from build123d import *

# Parameters (mm, degrees)
SKETCH1_R           = 3.175
BOSS_EXTRUDE1_DEPTH = 12.7
SKETCH2_R           = 5.08
BOSS_EXTRUDE2_DEPTH = 3.175
MOVE_FACE1_BY       = 0.250000008


with BuildPart() as part:
    # Sketch1 → Boss-Extrude1 (new body)
    with BuildSketch(Plane.XY):
        Circle(SKETCH1_R)
    extrude(amount=BOSS_EXTRUDE1_DEPTH)

    # Sketch2 → Boss-Extrude2 (add)
    with BuildSketch(Plane(origin=(0, 0, 0), x_dir=(-1, 0, 0), z_dir=(0, 0, -1))):
        Circle(SKETCH2_R)
    extrude(amount=BOSS_EXTRUDE2_DEPTH)

    # Move Face1: a curved face moved inward by 0.25
    add(Solid.thicken(part.faces().sort_by_distance((-3.175, 0, 6.35))[0], -MOVE_FACE1_BY), mode=Mode.SUBTRACT)


solid = part.part
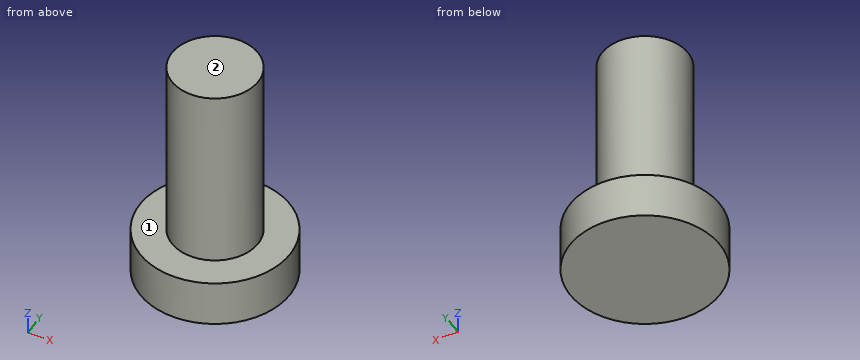
Geometry check sheet. Reference: the model listing, model coordinates, mm. Face numbers are marked on the shaded views. A direction names the side the tool comes from. Coordinates: 2 decimals unless noted, no trailing zeros. Loops run counter-clockwise (first coordinate to the right, second up) from the corner with the lowest first, then second, coordinate; pieces in that order, holes last. Notation, with made-up numbers: (62, 56.5) - (96, 56.5) arc R26 ccw to (96, 78.5) - close; hole circle Ø7 at (-7, 18). An arc over 180 degrees is marked (long way). Use one line per item in the form item = value. Start each with the question number.
Item 1: Section check D-D, the plane y = 3.5. Enter the section's corners in (x, z) (3 decimals), and give its area (3 significant figures).
Item 2: Tool access check on the marked faces 1 and 2. Record the directions out of +Z, -Z, +X, -X, +Y, -Y that give a thin tool (end or side, any length) a straight path to the whole face; none if there is none.
Item 3: Section check C-C, the plane z = 5.25. Enter the section's corners in (x, y) (3 decimals), and give its area (3 significant figures).
Item 4: Thickness scan on probe 1 along Z at (x, y) = (-0.25, 4) (3 decimals); probe 2 along X at (y, z) = (4, -1.25); probe 3 along Y at (x, z) = (2, 5.25). Record the ranges inside material, lowest first.
Item 5: Gauge pin test, flat ends, axial feed: pin 1 (6 mm diameter, centred on x = -0.5, z = 9, fed in from +Y) (3 decimals); pin 2 (5 mm diameter, centred on x = -3, z = 1.5, fed in from -Y); pin 3 (1.5 mm diameter, centred on x = 2.5, y = -3, fed in from +Z). Record the tip position at first contact, or that the pin passes through.
Item 6: Section check A-A, the plane x = 0. Enter the section's corners in (y, z) (3 decimals), and give its area (3 significant figures).
Computed:
q1.outline = (-3.682, -3.175) - (3.682, -3.175) - (3.682, 0) - (-3.682, 0) - close
q1.area = 23.4 mm2
q2.face_1 = +Z
q2.face_2 = +Z, +X, -X, +Y, -Y
q3.outline = circle Ø5.85 at (0, 0)
q3.area = 26.9 mm2
q4.probe_1 = -3.175 to 0
q4.probe_2 = -3.13 to 3.13
q4.probe_3 = -2.13 to 2.13
q5.pin_1 = 2.925
q5.pin_2 = -4.98
q5.pin_3 = 0
q6.outline = (-5.08, -3.175) - (5.08, -3.175) - (5.08, 0) - (2.925, 0) - (2.925, 12.7) - (-2.925, 12.7) - (-2.925, 0) - (-5.08, 0) - close
q6.area = 107 mm2
